The listing builds one solid part. Answer for the finished solid, in the listing's coordinates (mm). A direction names the side the tool comes from. Coordinates: 2 decimals unless noted, no trailing zeros. Write each loop counter-clockwise with the first axis right and the second up, starting at its lowest first coordinate (ties: lowest second). Pieces come first, ordered by that corner, then holes. Notation, with made-up numbers: M -29.75,5 L 2.25,5 A12 ccw 2.25,13 Z; hole C 30.25,43 d10. An arc over 180 degrees is marked long. Put each result on its own line as item: value. Start each with the question number.
```python
from build123d import *
from OCP.BRepAlgoAPI import BRepAlgoAPI_Cut
from OCP.TopTools import TopTools_ListOfShape

# Parameters (mm, degrees)
BOSS_EXTRUDE2_DEPTH          = 150
SKETCH4_W                    = 40
SKETCH4_H                    = 124.999999274
CUT_EXTRUDE4_DEPTH           = 20
SKETCH8_W                    = 50
SKETCH8_H                    = 124.997967802
CUT_EXTRUDE8_DEPTH           = 30
CUT_EXTRUDE10_DEPTH          = 231.489840965
CUT_EXTRUDE10_DEPTH_BACK     = 231.489840965
CUT_EXTRUDE11_DEPTH          = 225.566109405
CUT_EXTRUDE11_DEPTH_BACK     = 225.566109405
SKETCH11_W                   = 112.022201576
SKETCH11_H                   = 106.194456985
CUT_EXTRUDE12_DEPTH          = 55
SKETCH13_W                   = 40
SKETCH13_H                   = 124.999999274
CUT_EXTRUDE13_DEPTH          = 20
SKETCH14_W                   = 50
SKETCH14_H                   = 124.999999274
CUT_EXTRUDE15_DEPTH          = 30
CUT_EXTRUDE17_DEPTH          = 120
SKETCH17_W                   = 30
SKETCH17_H                   = 5.259472701
BOSS_EXTRUDE3_DEPTH          = 55
CUT_EXTRUDE18_DEPTH          = 225.566109405
CUT_EXTRUDE18_DEPTH_BACK     = 225.566109405
SKETCH20_R                   = 12
CUT_EXTRUDE_THIN2_DEPTH      = 244.166481024
CUT_EXTRUDE_THIN2_DEPTH_BACK = 244.166481024
SKETCH21_W                   = 50
SKETCH21_H                   = 219.250605911
SKETCH22_W                   = 4
SKETCH22_H                   = 160
BOSS_EXTRUDE4_DEPTH          = 5
SKETCH25_W                   = 30
SKETCH25_H                   = 57.6
BOSS_EXTRUDE5_DEPTH          = 18
SKETCH25_4_W                 = 24
SKETCH25_4_H                 = 51.6
CUT_EXTRUDE19_DEPTH          = 13
SKETCH26_W                   = 0.687822724
SKETCH26_H                   = 5.268229282
SKETCH26_H_2                 = 2.219145295
CUT_EXTRUDE21_DEPTH          = 1
CUT_EXTRUDE22_DEPTH          = 5
CUT_EXTRUDE22_DEPTH_BACK     = 5
SKETCH28_R                   = 0.75


with BuildPart() as part:
    # Sketch1 → Boss-Extrude2 (new body)
    with BuildSketch(Plane(origin=(0, 0, 0), x_dir=(0, 0, -1), z_dir=(1, 0, 0))):
        with BuildLine():
            Line((-37.52319824, 25.023509242), (-37.52319824, -99.976490758))
            Line((-37.52319824, -99.976490758), (122.47680176, -99.976490758))
            Line((122.47680176, -99.976490758), (122.47680176, 25.023509242))
            ThreePointArc((122.47680176, 25.023509242), (42.47680176, 105.023509242), (-37.52319824, 25.023509242))
        make_face()
    extrude(amount=BOSS_EXTRUDE2_DEPTH)

    # Sketch4 → Cut-Extrude4 (cut)
    with BuildSketch(Plane.XY.offset(37.52319824)):
        with Locations((20, -37.476491121)):
            Rectangle(SKETCH4_W, SKETCH4_H)
    extrude(amount=-CUT_EXTRUDE4_DEPTH, mode=Mode.SUBTRACT)

    # Sketch8 → Cut-Extrude8 (cut)
    with BuildSketch(Plane.XY.offset(37.52319824)):
        with Locations((65, -37.477506857)):
            Rectangle(SKETCH8_W, SKETCH8_H)
    extrude(amount=-CUT_EXTRUDE8_DEPTH, mode=Mode.SUBTRACT)

    # Sketch9 → Cut-Extrude10 (cut, two sides: drawn at the far end of the back side and taken through both)
    with BuildSketch(Plane.XZ.offset(-25.023508516).offset(-CUT_EXTRUDE10_DEPTH_BACK)):
        Polygon((0, 37.52319824), (0, 17.52319824), (40, 17.52319824), (40, 7.52319824), (90, 7.52319824), (90, 37.52319824), align=None)
    extrude(amount=CUT_EXTRUDE10_DEPTH + CUT_EXTRUDE10_DEPTH_BACK, mode=Mode.SUBTRACT)

    # Sketch11 → Cut-Extrude11 (cut, two sides: drawn at the far end of the back side and taken through both)
    with BuildSketch(Plane.XY.offset(7.52319824).offset(-CUT_EXTRUDE11_DEPTH_BACK)):
        with Locations((33.988899212, 78.120737735)):
            Rectangle(SKETCH11_W, SKETCH11_H)
    extrude(amount=CUT_EXTRUDE11_DEPTH + CUT_EXTRUDE11_DEPTH_BACK, mode=Mode.SUBTRACT)

    # Sketch12 → Cut-Extrude12 (cut)
    with BuildSketch(Plane(origin=(150, 0, 0), x_dir=(0, 0, -1), z_dir=(1, 0, 0))):
        with BuildLine():
            Line((117.47680176, 25.023509242), (117.47680176, -94.976490758))
            Line((117.47680176, -94.976490758), (-32.52319824, -94.976490758))
            Line((-32.52319824, -94.976490758), (-32.52319824, 25.023509242))
            ThreePointArc((-32.52319824, 25.023509242), (42.47680176, 100.023509242), (117.47680176, 25.023509242))
        make_face()
    extrude(amount=-CUT_EXTRUDE12_DEPTH, mode=Mode.SUBTRACT)


with BuildPart() as cut_extrude13_tool:
    # Sketch13 → Cut-Extrude13 (new body)
    with BuildSketch(Plane(origin=(0, 0, -122.47680176), x_dir=(-1, 0, 0), z_dir=(0, 0, -1))):
        with Locations((-20, -37.476490395)):
            Rectangle(SKETCH13_W, SKETCH13_H)
    extrude(amount=-CUT_EXTRUDE13_DEPTH)


with BuildPart() as part_1:
    add(part.part)

    # Cut-Extrude13: cut by cut_extrude13_tool, with a tolerance
    cut_extrude13_stock = TopTools_ListOfShape()
    cut_extrude13_stock.Append(part_1.part.wrapped)
    cut_extrude13_tools = TopTools_ListOfShape()
    cut_extrude13_tools.Append(cut_extrude13_tool.part.wrapped)
    cut_extrude13_cut = BRepAlgoAPI_Cut()
    cut_extrude13_cut.SetArguments(cut_extrude13_stock)
    cut_extrude13_cut.SetTools(cut_extrude13_tools)
    cut_extrude13_cut.SetFuzzyValue(0.00001)
    cut_extrude13_cut.Build()
    add(Compound.cast(cut_extrude13_cut.Shape()).solids(), mode=Mode.REPLACE)


with BuildPart() as cut_extrude15_tool:
    # Sketch14 → Cut-Extrude15 (new body)
    with BuildSketch(Plane(origin=(0, 0, -122.47680176), x_dir=(-1, 0, 0), z_dir=(0, 0, -1))):
        with Locations((-65, -37.476490395)):
            Rectangle(SKETCH14_W, SKETCH14_H)
    extrude(amount=-CUT_EXTRUDE15_DEPTH)


with BuildPart() as part_2:
    add(part_1.part)

    # Cut-Extrude15: cut by cut_extrude15_tool, with a tolerance
    cut_extrude15_stock = TopTools_ListOfShape()
    cut_extrude15_stock.Append(part_2.part.wrapped)
    cut_extrude15_tools = TopTools_ListOfShape()
    cut_extrude15_tools.Append(cut_extrude15_tool.part.wrapped)
    cut_extrude15_cut = BRepAlgoAPI_Cut()
    cut_extrude15_cut.SetArguments(cut_extrude15_stock)
    cut_extrude15_cut.SetTools(cut_extrude15_tools)
    cut_extrude15_cut.SetFuzzyValue(0.00001)
    cut_extrude15_cut.Build()
    add(Compound.cast(cut_extrude15_cut.Shape()).solids(), mode=Mode.REPLACE)

    # Sketch16 → Cut-Extrude17 (cut)
    with BuildSketch(Plane.XZ.offset(99.976490758)):
        Polygon((95, -87.47680176), (95, -117.47680176), (145, -117.47680176), (145, 32.52319824), (95, 32.52319824), (95, 2.52319824), (35, 2.52319824), (35, 12.52319824), (5, 12.52319824), (5, -97.47680176), (35, -97.47680176), (35, -87.47680176), align=None)
    extrude(amount=-CUT_EXTRUDE17_DEPTH, mode=Mode.SUBTRACT)

    # Sketch17 → Boss-Extrude3 (add)
    with BuildSketch(Plane(origin=(95, 0, 0), x_dir=(0, 0, -1), z_dir=(1, 0, 0))):
        with Locations((-17.52319824, 22.653245593)):
            Rectangle(SKETCH17_W, SKETCH17_H)
    extrude(amount=BOSS_EXTRUDE3_DEPTH)

    # Sketch20 → Cut-Extrude18 (cut, two sides: drawn at the far end of the back side and taken through both)
    with BuildSketch(Plane.XY.offset(7.52319824).offset(-CUT_EXTRUDE18_DEPTH_BACK)):
        with Locations(Location((26.097811204, -32.450551048, 0), (0, 0, 317.88916676))):
            Circle(SKETCH20_R)
    extrude(amount=CUT_EXTRUDE18_DEPTH + CUT_EXTRUDE18_DEPTH_BACK, mode=Mode.SUBTRACT)

    # Sketch21 → Cut-Extrude-Thin2 (cut, two sides: drawn at the far end of the back side and taken through both)
    with BuildSketch(Plane(origin=(0, 0, -122.47680176), x_dir=(-1, 0, 0), z_dir=(0, 0, -1)).offset(-CUT_EXTRUDE_THIN2_DEPTH_BACK)):
        with Locations((-145.127265144, 6.610737582)):
            Rectangle(SKETCH21_W, SKETCH21_H)
    extrude(amount=CUT_EXTRUDE_THIN2_DEPTH + CUT_EXTRUDE_THIN2_DEPTH_BACK, mode=Mode.SUBTRACT)

    # Sketch22 → Boss-Extrude4 (add)
    with BuildSketch(Plane.XZ.offset(99.976490758)):
        with Locations((118.127265144, -42.47680176)):
            Rectangle(SKETCH22_W, SKETCH22_H)
    extrude(amount=-BOSS_EXTRUDE4_DEPTH)

    # Sketch25 → Boss-Extrude5 (add)
    with BuildSketch(Plane.ZY):
        with Locations((-42.190239987, -37.637506258)):
            Rectangle(SKETCH25_W, SKETCH25_H)
    extrude(amount=-BOSS_EXTRUDE5_DEPTH)

    # Sketch25_4 → Cut-Extrude19 (cut)
    with BuildSketch(Plane.ZY):
        with Locations((-42.190239987, -37.637506258)):
            Rectangle(SKETCH25_4_W, SKETCH25_4_H)
    extrude(amount=-CUT_EXTRUDE19_DEPTH, mode=Mode.SUBTRACT)

    # Sketch26 → Cut-Extrude21 (cut)
    with BuildSketch(Plane(origin=(0, -63.437506258, 0), x_dir=(1, 0, 0), z_dir=(0, 1, 0))):
        with Locations((0.643930004, 33.960425166)):
            Rectangle(SKETCH26_W, SKETCH26_H)
        with Locations((0.643930004, 53.134905876)):
            Rectangle(SKETCH26_W, SKETCH26_H_2)
    extrude(amount=-CUT_EXTRUDE21_DEPTH, mode=Mode.SUBTRACT)

    # Sketch28 → Cut-Extrude22 (cut, two sides: drawn at the far end of the back side and taken through both)
    with BuildSketch(Plane(origin=(0, -8.837506258, 0), x_dir=(1, 0, 0), z_dir=(0, 1, 0)).offset(-CUT_EXTRUDE22_DEPTH_BACK)):
        with Locations(Location((10.149113082, 44.540239987, 0), (0, 0, 270))):
            Circle(SKETCH28_R)
        with Locations(Location((10.149113082, 39.840239987, 0), (0, 0, 270))):
            Circle(SKETCH28_R)
    extrude(amount=CUT_EXTRUDE22_DEPTH + CUT_EXTRUDE22_DEPTH_BACK, mode=Mode.SUBTRACT)


solid = part_2.part
```
1) A cutting plane is placed at C-C on z = -49. Write down the section's boundary in (x, y).
2) Determine the mould class of faces 6 (the face through (104.853, 105.004, -44.236)), 7 (the face through (11, -37, -102.477)), 8 (the face through (37.006, -37.452, 13.252)) for opening direction Y: +Y half, -Y half, draft (parallel to the pull), parting line (faces both ways), or undercut.
3) Straight lines are drawn through the part: probe 1 along Z at (x, y) = (92, -15); probe 2 along Z at (x, y) = (6, -39); probe 3 along Z at (x, y) = (40.5, 11). For each, find the intervals that lie inside material, in ascending order.
4) Given pin 1 Ø1.4 at (x, z) = (10.15, -39.84) entering from +Y; pin 2 Ø8 at (x, y) = (49, -69.5) entering from +Z; pin 3 Ø1.1 at (y, z) = (-63.5, -35) entering from +X, each flat-ended and moving along its own axis, determine where each tip first touches the part or whether it passes through.
5) For faces 1 (the face through (37.006, -37.452, -98.415)), 2 (the face through (11, -37, 17.523)), 3 (the face through (13, -37, -42)), 4 (the face through (16, -41, -97.477)), 5 (the face through (90, 27, -44)), determine the directions among +Z, -Z, +X, -X, +Y, -Y from which every point of the face is accessible in a straight line to the end or side of a thin tool.
6) A cutting plane is placed at D-D on x = 30. Write down the section's boundary in (y, z).
7) A cutting plane is placed at B-B on y = -75. Write down the section's boundary in (x, z).
Answers follow:
1. outline: M 0,-99.98 L 5,-99.98 L 5,-66.44 L 18,-66.44 L 18,-8.84 L 5,-8.84 L 5,20.02 L 95,20.02 L 95,99.74 L 120.13,99.74 L 120.13,104.76 L 90,104.76 L 90,25.02 L 0,25.02 L 0,-11.84 L 13,-11.84 L 13,-63.44 L 0,-63.44 Z; M 116.13,-99.98 L 120.13,-99.98 L 120.13,-94.98 L 116.13,-94.98 Z
2. face 6: +Y half
2. face 7: draft
2. face 8: undercut
3. probe 1: z = -122.48 to -87.48, 2.52 to 37.52
3. probe 2: z = -102.48 to -97.48, -57.19 to -54.19, -30.19 to -27.19, 12.52 to 17.52
3. probe 3: z = -92.48 to -87.48, 2.52 to 7.52
4. pin 1: stops at y = 25.02
4. pin 2: stops at z = 7.52
4. pin 3: stops at x = 18
5. face 1: -Z
5. face 2: +Z, -X, +Y, -Y
5. face 3: -X
5. face 4: -Y
5. face 5: +Y
6. outline: M -99.98,-102.48 L -43.8,-102.48 L -43.8,-97.48 L -99.98,-97.48 Z; M -99.98,12.52 L -43.8,12.52 L -43.8,17.52 L -99.98,17.52 Z; M -21.1,-102.48 L 25.02,-102.48 L 25.02,17.52 L -21.1,17.52 L -21.1,12.52 L 20.02,12.52 L 20.02,-97.48 L -21.1,-97.48 Z
7. outline: M 0,-102.48 L 40,-102.48 L 40,-92.48 L 90,-92.48 L 90,-122.48 L 120.13,-122.48 L 120.13,-117.48 L 95,-117.48 L 95,-87.48 L 35,-87.48 L 35,-97.48 L 5,-97.48 L 5,12.52 L 35,12.52 L 35,2.52 L 95,2.52 L 95,32.52 L 120.13,32.52 L 120.13,37.52 L 90,37.52 L 90,7.52 L 40,7.52 L 40,17.52 L 0,17.52 Z
